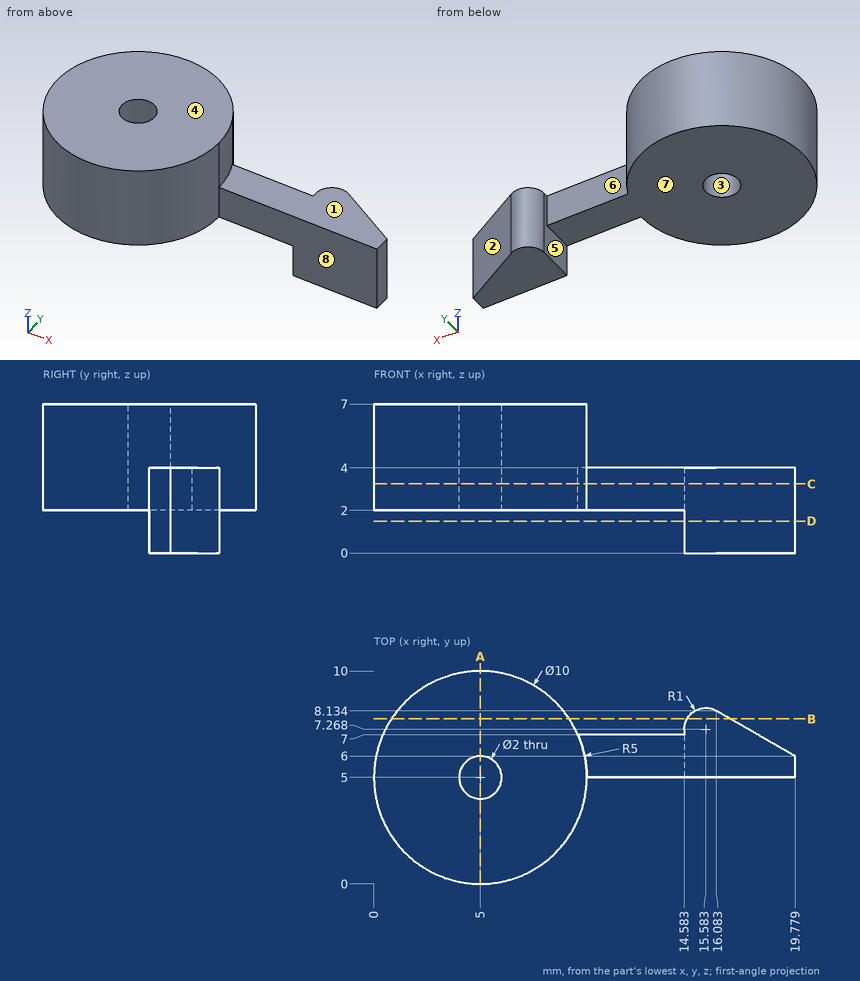
Part print with two shaded views. Sizes in mm from the minimum x, y, z corner. A direction names the side the tool comes from. Coordinates: 2 decimals unless noted, no trailing zeros. Order: outer loops, then holes, each group sorted by start corner. A loop starts at its lowest first (then second) coordinate and runs counter-clockwise, first axis right, second up. Notation, with made-up numbers: M 81.25,-19 L 131.25,-19 A30 ccw 131.25,15 Z; hole C 11.5,-26.5 d7. An arc over 180 degrees is marked long. One line per question, with ' | ' between items. Start each with the question number.
1. Cut at B-B (y = 7.75). Write the cut outline in (x, z) (1 decimal).
2. Wall check: line 1 along X through (y, z) = (5, 4.4); line 2 along Z through (x, y) = (1.25, 7.75). Give the ranges that are in metal, low to high. Write a range as [from, to].
3. Cut at C-C (z = 3.25). Write the cut outline in (x, y).
4. Cut at D-D (z = 1.5). Write the cut outline in (x, y).
5. Tool access for the marked faces 4, 5, 6, 7 and 8: list every direction of +Z, -Z, +X, -X, +Y, -Y with a clear straight run to the whole face (end or side of a thin tool).
6. Mould opens along X. For the marked faces 1, 2 and 3 say: +X half, -X half, draft (parallel to the pull), parting line (faces both ways), or undercut.
7. Cut at A-A (x = 5). Write the cut outline in (y, z).
8. Flat gauge pins, fed straight in: P1, Ø1.1, axis at y = 6, z = 1, coming from the -X side; P2, Ø3.5, axis at x = 12, y = 6.5, coming from the +Z side; P3, Ø1.6, axis at x = 5, y = 5, coming from the +Z side; P4, Ø1, axis at x = 7.5, z = 4.5, coming from the -Y side. Where does each tip first touch, or does it go through?
The answers:
1) outline: M 0.8,2 L 9.2,2 L 9.2,7 L 0.8,7 Z; M 14.7,0 L 16.7,0 L 16.7,4 L 14.7,4 Z
2) line 1: x = [0, 4], [6, 10] | line 2: z = [2, 7]
3) outline: M 9.58,7 A5 ccw long 10,5 L 19.78,5 L 19.78,6 L 16.08,8.13 A1 ccw 14.58,7.27 L 14.58,7 Z; hole C 5,5 d2
4) outline: M 14.58,5 L 19.78,5 L 19.78,6 L 16.08,8.13 A1 ccw 14.58,7.27 Z
5) face 4: +Z, +X, -X, +Y, -Y | face 5: -Z, +Y | face 6: +Z, -Z, +Y | face 7: -Z, -X, +Y, -Y | face 8: +Z, -Z, +X, -Y
6) face 1: draft | face 2: +X half | face 3: undercut
7) outline: M 0,2 L 4,2 L 4,7 L 0,7 Z; M 6,2 L 10,2 L 10,7 L 6,7 Z
8) P1: stops at x = 14.58 | P2: stops at z = 4 | P3: passes through | P4: stops at y = 0.42
